```python
from build123d import *

# Parameters (mm, degrees)
F0_W     = 30
F0_H     = 80
F1_DEPTH = 30
F2_R     = 5
F4_DEPTH = 30
F5_R     = 5
F6_DEPTH = 30


with BuildPart() as f1:
    # F0 (on Top) → F1 (new body)
    with BuildSketch(Plane.XY):
        Rectangle(F0_W, F0_H)
    extrude(amount=F1_DEPTH)

    # F2
    f2_edges = [f1.edges().sort_by_distance(p)[0] for p in [
        (15, 40, 15),
        (-15, 40, 15),
        (-15, -40, 15),
        (15, -40, 15),
    ]]
    fillet(f2_edges, radius=F2_R)

    # F3 (on face) → F4 (cut)
    with BuildSketch(Plane.XY.offset(30)):
        with BuildLine():
            ThreePointArc((13, 35), (12.12132, 37.12132), (10, 38))
            Line((10, 38), (-10, 38))
            ThreePointArc((-10, 38), (-12.12132, 37.12132), (-13, 35))
            Line((-13, 35), (-13, -35))
            ThreePointArc((-13, -35), (-12.12132, -37.12132), (-10, -38))
            Line((-10, -38), (10, -38))
            ThreePointArc((10, -38), (12.12132, -37.12132), (13, -35))
            Line((13, -35), (13, 35))
        make_face()
    extrude(amount=-F4_DEPTH, mode=Mode.SUBTRACT)

    # F5 (on face) → F6 (cut)
    with BuildSketch(Plane.YZ.offset(15)):
        with Locations((0, 15)):
            Circle(F5_R)
    extrude(amount=-F6_DEPTH, mode=Mode.SUBTRACT)


solid = f1.part
```
Check sheet for the modelled part. Datum: model origin and axes. Units: mm. A direction names the side the tool comes from. Coordinates: 2 decimals unless noted, no trailing zeros. Loops run counter-clockwise (first coordinate to the right, second up) from the corner with the lowest first, then second, coordinate; pieces in that order, holes last.
1) Sectioned sample at A-A (y = 11). Record the boundary of the cut face in (x, z), and give its area (3 significant figures).
2) Sectioned sample at B-B (z = 15). Record the boundary of the cut face in (x, y), and give its area (3 significant figures).
3) Sectioned sample at D-D (y = 0). Record the boundary of the cut face in (x, z).
4) Material ranges on probe 1 along X at (y, z) = (17.5, 21); probe 2 along Y at (x, z) = (0.5, 6.75); probe 3 along Z at (x, y) = (-13.5, 0), recorded low to high.
5) Sectioned sample at C-C (x = -9.25). Record the boundary of the cut face in (y, z).
6) Release check for a two-part mould opening along Z. For faces 1 (the face through (-12.1, 37.14, 15.21)), 2 (the face through (-13.99, -1.08, 10.12)), 3 (the face through (-13.4, 0.2, 30)) record: released by +Z, released by -Z, zero draft, split by the parting line, or undercut.
7) Access from +Z, -Z, +X, -X, +Y, -Y to the whole of each face (thin tool, end or side, straight path). Record for faces 4 (the face through (13, 0, 22)), 5 (the face through (14.01, -1.08, 10.12)).
Check sheet entries:
1. outline: (-15, 0) - (-13, 0) - (-13, 30) - (-15, 30) - close; (13, 0) - (15, 0) - (15, 30) - (13, 30) - close
1. area: 120 mm2
2. outline: (-15, -35) arc R5 ccw to (-10, -40) - (10, -40) arc R5 ccw to (15, -35) - (15, -5) - (13, -5) - (13, -35) arc R3 cw to (10, -38) - (-10, -38) arc R3 cw to (-13, -35) - (-13, -5) - (-15, -5) - close; (-15, 5) - (-13, 5) - (-13, 35) arc R3 cw to (-10, 38) - (10, 38) arc R3 cw to (13, 35) - (13, 5) - (15, 5) - (15, 35) arc R5 ccw to (10, 40) - (-10, 40) arc R5 ccw to (-15, 35) - close
2. area: 370 mm2
3. outline: (-15, 0) - (-13, 0) - (-13, 10) - (-15, 10) - close; (-15, 20) - (-13, 20) - (-13, 30) - (-15, 30) - close; (13, 0) - (15, 0) - (15, 10) - (13, 10) - close; (13, 20) - (15, 20) - (15, 30) - (13, 30) - close
4. probe 1: x = -15 to -13, 13 to 15
4. probe 2: y = -40 to -38, 38 to 40
4. probe 3: z = 0 to 10, 20 to 30
5. outline: (-40, 0) - (-38, 0) - (-38, 30) - (-40, 30) - close; (38, 0) - (40, 0) - (40, 30) - (38, 30) - close
6. face 1: zero draft
6. face 2: undercut
6. face 3: released by +Z
7. face 4: +Z, -Z
7. face 5: +X, -X
